The listing builds one solid part. Answer for the finished solid, in the listing's coordinates (mm). A direction names the side the tool comes from. Round coordinates to 2 decimals unless told otherwise and drop trailing zeros. Write each loop counter-clockwise with the first axis right and the second up, starting at its lowest first coordinate (ties: lowest second). Pieces come first, ordered by that corner, then holes. Notation, with made-up numbers: M 32,39 L 63,39 A14 cw 63,49 Z; hole C 44.5,-5.75 d8. An arc over 180 degrees is marked long. Write each question's results on one line, items separated by ' | '.
from build123d import *

# Parameters (mm, degrees)
BOSS_EXTRUDE1_DEPTH             = 8.5
TAP_DRILL_FOR_M4X0_7_TAP1_D     = 4
TAP_DRILL_FOR_M4X0_7_TAP1_DEPTH = 5.298278762
TAP_DRILL_FOR_M4X0_7_TAP1_TIP   = 1.201721238
CUT_EXTRUDE1_DEPTH              = 17.980360556
CUT_EXTRUDE1_DEPTH_BACK         = 17.980360556
SKETCH5_R                       = 3


with BuildPart() as part:
    # Sketch1 → Boss-Extrude1 (new, symmetric)
    with BuildSketch(Plane(origin=(0, 0, 0), x_dir=(1, 0, 0), z_dir=(0, 1, 0))):
        with BuildLine():
            Line((-8, 7), (-8, 4.5))
            Line((-8, 4.5), (8, 4.5))
            Line((8, 4.5), (8, 7))
            Line((8, 7), (10.866583853, 7))
            ThreePointArc((10.866583853, 7), (12.926045204, 0), (10.866583853, -7))
            Line((10.866583853, -7), (8, -7))
            Line((8, -7), (8, -4.5))
            Line((8, -4.5), (-8, -4.5))
            Line((-8, -4.5), (-8, -7))
            Line((-8, -7), (-10.866583853, -7))
            ThreePointArc((-10.866583853, -7), (-12.926045204, 0), (-10.866583853, 7))
            Line((-10.866583853, 7), (-8, 7))
        make_face()
    extrude(amount=BOSS_EXTRUDE1_DEPTH, both=True)

    # Tap Drill for M4x0.7 Tap1
    with Locations(Plane(origin=(0, 8.5, 0), x_dir=(1, 0, 0), z_dir=(0, 1, 0))):
        with Locations((0, 0)):
            Hole(TAP_DRILL_FOR_M4X0_7_TAP1_D / 2, depth=TAP_DRILL_FOR_M4X0_7_TAP1_DEPTH)
            with Locations((0, 0, -(TAP_DRILL_FOR_M4X0_7_TAP1_DEPTH + TAP_DRILL_FOR_M4X0_7_TAP1_TIP / 2))):  # 118° drill point
                Cone(0, TAP_DRILL_FOR_M4X0_7_TAP1_D / 2, TAP_DRILL_FOR_M4X0_7_TAP1_TIP, mode=Mode.SUBTRACT)

    # Sketch5 → Cut-Extrude1 (cut, two sides: drawn at the far end of the back side and taken through both)
    with BuildSketch(Plane.XY.offset(-CUT_EXTRUDE1_DEPTH_BACK)):
        with Locations((0, -1.5)):
            Circle(SKETCH5_R)
    extrude(amount=CUT_EXTRUDE1_DEPTH + CUT_EXTRUDE1_DEPTH_BACK, mode=Mode.SUBTRACT)


solid = part.part
1) Section D-D (x = 6) is taken. Determine the outline of the cut face in (y, z), then the cut area to 3 significant figures.
Return value:
outline: M -8.5,-4.5 L 8.5,-4.5 L 8.5,4.5 L -8.5,4.5 Z | area: 153 mm²
2) Section B-B (z = -5.5) is taken. Determine the outline of the cut face in (x, y), then the cut area to 3 significant figures.
Return value:
outline: M -11.7,-8.5 L -8,-8.5 L -8,8.5 L -11.7,8.5 Z; M 8,-8.5 L 11.7,-8.5 L 11.7,8.5 L 8,8.5 Z | area: 126 mm²
3) Section C-C (z = 4) is taken. Determine the outline of the cut face in (x, y).
Return value:
outline: M -12.29,-8.5 L 12.29,-8.5 L 12.29,8.5 L -12.29,8.5 Z; hole C 0,-1.5 d6
4) Section A-A (y = -1.5) is taken. Determine the outline of the cut face in (x, z).
Return value:
outline: M -10.87,-7 L -8,-7 L -8,-4.5 L -3,-4.5 L -3,4.5 L -8,4.5 L -8,7 L -10.87,7 A12.93 ccw Z; M 3,-4.5 L 8,-4.5 L 8,-7 L 10.87,-7 A12.93 ccw 10.87,7 L 8,7 L 8,4.5 L 3,4.5 Z
5) A tool of negligible diameter and unlimited length cuts with its end or side. For faces 1 (the face through (8, 0, -6)), 2 (the face through (8, 0, 6)), 3 (the face through (0, 6, 2)), from which of +Z, -Z, +X, -X, +Y, -Y can it reach the whole face along a straight path? Write none if from no direction.
Return value:
face 1: -Z, +Y, -Y | face 2: +Z, +Y, -Y | face 3: +Y
6) Find the intervals of material crossed by line 1 (Z direction, x = 0, y = 7); line 2 (Y direction, x = 0, z = 0.25); line 3 (Z direction, x = 3.25, y = -2), in increasing order.
Return value:
line 1: -4.5 to -2, 2 to 4.5 | line 2: -8.5 to -4.5, 1.5 to 2.15 | line 3: -4.5 to 4.5
7) Each of these flat-tipped pins is pushed along its axis until it touches: pin 1 (6 mm diameter, centred on y = 5, z = 4, fed in from -X); pin 2 (8 mm diameter, centred on x = -3.5, y = 3, fed in from -Z); pin 3 (1.2 mm diameter, centred on y = 1.5, z = -5.5, fed in from +X). Where does it stop, or does it pass through?
Return value:
pin 1: x = -12.89 | pin 2: z = -4.5 | pin 3: x = 11.96
8) The mould has two halves that part along Y. Classify faces 4 (the face through (-3, 8.5, 0)), 5 (the face through (-8, 0, -6)), 6 (the face through (-3, -1.4, -0.1)): +Y half, -Y half, draft (parallel to the pull), parting line (faces both ways), or undercut.
Return value:
face 4: +Y half | face 5: draft | face 6: undercut
